Could you check a few things on this drawing? It's one solid part, dimensions in mm from its lowest x, y, z. A direction names the side the tool comes from. Coordinates: 2 decimals unless noted, no trailing zeros. Order: outer loops, then holes, each group sorted by start corner. A loop starts at its lowest first (then second) coordinate and runs counter-clockwise, first axis right, second up. Notation, with made-up numbers: (78.25, 69.5) -> (84.25, 69.5) arc R20 ccw to (84.25, 73.5) -> close; hole circle Ø6 at (46.25, -17). An arc over 180 degrees is marked (long way). Use a Markdown table: item, result. Add a question column.
1. Suppose I cut it at A-A, the plane z = 0.7. State how many separate pieces and enclosed holes the cut face has, then the cut area to 3 significant figures.
2. Suppose I cut it at C-C, the plane x = 11. List the corners of the cut face in (y, z) for me, then the cut area to 3 significant figures.
3. We'd pull the mould along Y, two halves only. Please class the marked faces 1, 2, 3 and 4: pulls with the +Y half, pulls with the -Y half, needs draft (parallel to the pull), parting line crosses it, or undercut.
4. For the marked faces 5, 6 and 7, which set-ups out of +Z, -Z, +X, -X, +Y, -Y let a thin tool reach every point of the face, with its end or its side?
5. Suppose I cut it at B-B, the plane y = 16. List the corners of the cut face in (x, z) for me.
6. Suppose I cut it at D-D, the plane x = 6. List the corners of the cut face in (y, z) for me.
7. If I drill on line 1 along Y through (x, z) = (20.5, 1.35); line 2 along Y through (x, z) = (20.5, 0.75); line 3 along X through (y, z) = (35, 1.05), over which ranges is the centre line in solid material (lowest first)? Write a range as from..to.
8. For pin 1 Ø2.5 at (x, y) = (20.5, 37) entering from -Z; pin 2 Ø1 at (x, z) = (8.5, 0.5) entering from +Y; pin 3 Ø1 at (x, z) = (35.5, 1.5) entering from -Y; pin 4 Ø1 at (y, z) = (19, 1) entering from +X, each with a flat end and sliding along its axis, tell me the tip position at first contact or that it passes through.
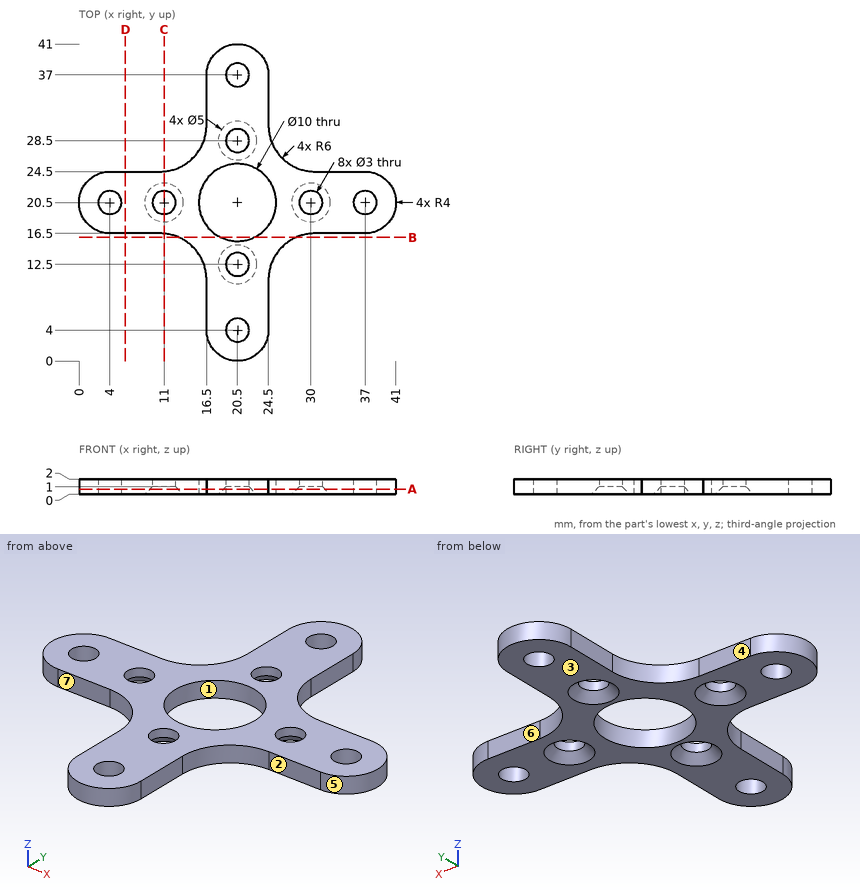
Worked out:
| question | item | result |
|---|---|---|
| 1 | separate pieces | 1 |
| 1 | enclosed holes | 9 |
| 1 | area | 448 mm² |
| 2 | outline | (16.48, 0) -> (18, 0) -> (19, 1) -> (19, 2) -> (16.48, 2) -> close; (22, 1) -> (23, 0) -> (24.52, 0) -> (24.52, 2) -> (22, 2) -> close |
| 2 | area | 9.08 mm² |
| 3 | face 1 | undercut |
| 3 | face 2 | pulls with the -Y half |
| 3 | face 3 | needs draft |
| 3 | face 4 | pulls with the +Y half |
| 4 | face 5 | +Z, -Z, +X |
| 4 | face 6 | +Z, -Z, +X, +Y |
| 4 | face 7 | +Z, -Z, -X, -Y |
| 5 | outline | (12.9, 0) -> (18.32, 0) -> (18.32, 2) -> (12.9, 2) -> close; (22.68, 0) -> (28.1, 0) -> (28.1, 2) -> (22.68, 2) -> close |
| 6 | outline | (16.5, 0) -> (24.5, 0) -> (24.5, 2) -> (16.5, 2) -> close |
| 7 | line 1 | y = 0..2.5, 5.5..11, 14..15.5, 25.5..27, 30..35.5, 38.5..41 |
| 7 | line 2 | y = 0..2.5, 5.5..10.75, 14.25..15.5, 25.5..26.75, 30.25..35.5, 38.5..41 |
| 7 | line 3 | x = 16.5..24.5 |
| 8 | pin 1 | passes through |
| 8 | pin 2 | stops at y = 24.5 |
| 8 | pin 3 | stops at y = 16.5 |
| 8 | pin 4 | stops at x = 40.87 |
